Model file for the job. Use its own axes, mm. Give positions to 0.01 mm unless a question says otherwise; leave off trailing zeros. Write each loop counter-clockwise with the first axis right and the second up, starting at its lowest first coordinate (ties: lowest second). Pieces come first, ordered by that corner, then holes.
```python
from build123d import *

# Parameters (mm, degrees)
SKETCH1_R           = 50
SKETCH1_R_2         = 38
SKETCH1_R_3         = 2.5
BOSS_EXTRUDE1_DEPTH = 2.5
CHAMFER1_SIZE       = 1


with BuildPart() as part:
    # Sketch1 → Boss-Extrude1 (new body)
    with BuildSketch(Plane(origin=(0, 0, 0), x_dir=(0, 0, -1), z_dir=(1, 0, 0))):
        Circle(SKETCH1_R)
        Circle(SKETCH1_R_2, mode=Mode.SUBTRACT)
        with Locations((0, 45)):
            Circle(SKETCH1_R_3, mode=Mode.SUBTRACT)
        with Locations((45, 0)):
            Circle(SKETCH1_R_3, mode=Mode.SUBTRACT)
        with Locations((0, -45)):
            Circle(SKETCH1_R_3, mode=Mode.SUBTRACT)
        with Locations((-45, 0)):
            Circle(SKETCH1_R_3, mode=Mode.SUBTRACT)
    extrude(amount=BOSS_EXTRUDE1_DEPTH)

    # Chamfer1
    chamfer1_edges = [part.edges().sort_by_distance(p)[0] for p in [
        (2.5, 0, -42.5),
        (2.5, -45, 2.5),
        (2.5, 0, 47.5),
        (2.5, 0, 50),
        (2.5, 0, 38),
        (2.5, 45, 2.5),
    ]]
    chamfer(chamfer1_edges, length=CHAMFER1_SIZE)


solid = part.part
```
1. Pull direction Z, two halves, no side cores. Call faces 1 (the flat face through (0, -18, 34)), 2 (the conical face through (2, 45, 3)), 3 (the cylindrical face through (0.74, 15.02, -47.69)): +Z half, -Z half, draft (parallel to the pull), parting line (faces both ways), or undercut.
Calculated:
face 1: draft
face 2: undercut
face 3: parting line
2. Slice it at A-A, the plane z = 0. Write the cut outline in (x, y).
Calculated:
outline: (0, -50) - (1.5, -50) - (2.5, -49) - (2.5, -48.5) - (1.5, -47.5) - (0, -47.5) - close; (0, -42.5) - (1.5, -42.5) - (2.5, -41.5) - (2.5, -39) - (1.5, -38) - (0, -38) - close; (0, 38) - (1.5, 38) - (2.5, 39) - (2.5, 41.5) - (1.5, 42.5) - (0, 42.5) - close; (0, 47.5) - (1.5, 47.5) - (2.5, 48.5) - (2.5, 49) - (1.5, 50) - (0, 50) - close
3. Pin check, flat tips, straight feed: P1, Ø6.5, axis at y = -45, z = 0, coming from the -X side; P2, Ø6.5, axis at y = 0, z = -45, coming from the +X side. Stop position of each tip, or through.
Calculated:
P1: stops at x = 0
P2: stops at x = 2.25
4. Probe probe 1 along Y at (x, z) = (0.8, 0); probe 2 along Z at (x, y) = (0.85, -44); probe 3 along Z at (x, y) = (0.95, 15). List the from-to ranges inside material, lowest first.
Calculated:
probe 1: y = -50 to -47.5, -42.5 to -38, 38 to 42.5, 47.5 to 50
probe 2: z = -23.75 to -2.29, 2.29 to 23.75
probe 3: z = -47.7 to -34.91, 34.91 to 47.7
5. Slice it at C-C, the plane x = 0.8. Write the cut outline in (y, z).
Calculated:
outline: circle Ø100 at (0, 0); hole circle Ø5 at (-45, 0); hole circle Ø76 at (0, 0); hole circle Ø5 at (0, -45); hole circle Ø5 at (0, 45); hole circle Ø5 at (45, 0)
